Check sheet for the modelled part. Datum: model origin and axes. Units: mm. Face numbers are marked on the shaded views. A direction names the side the tool comes from. Give positions to 0.01 mm unless a question says otherwise; leave off trailing zeros. Loops run counter-clockwise (first coordinate to the right, second up) from the corner with the lowest first, then second, coordinate; pieces in that order, holes last. Notation, with made-up numbers: M 20,-1.5 L 54,-1.5 A17 ccw 54,8.5 Z; hole C -5,21.5 d10. An arc over 180 degrees is marked long. Use one line per item in the form item = value.
Autodesk Inventor part; units mm, degrees
ref_plane "Work Plane1" through (30.1625, 0, 0) normal (0, 0, -1) x (1, 0, 0)
ref_plane "YZ Plane" through (0, 0, 0) normal (1, 0, 0) x (0, 1, 0)
ref_plane "XZ Plane" through (0, 0, 0) normal (0, 1, 0) x (-1, 0, 0)
sketch "Sketch1" plane through (0, 0, 0) normal (0, 0, 1) x (1, 0, 0)
  line L0 (-3.3, 0) -> (50, 0)
  line L1 (50, 0) -> (50, 2.5)
  line L2 (50, 2.5) -> (12, 2.5)
  line L3 (12, 2.5) -> (11.5091, 2.2835)
  line L4 (11.5091, 2.2835) -> (0, 2.2835)
  line L5 (0, 2.2835) -> (0, 4.25)
  line L6 (-13.96, 0) -> (60.66, 0)
  line L7 (0, -0.85) -> (0, 5.1)
  line L8 (-3.3, 0) -> (-3.3, 3.9613)
  line L9 (0, 4.25) -> (-3.3, 3.9613)
  line L10 (12, 2.5) -> (0, 2.5) construction
  dimension "d0" = 50
  dimension "d1" = 38
  dimension "d2" = 0.4909
  dimension "d3" = 3.3
  dimension "d4" = 5
  dimension "d5" = 4.567
  dimension "d9" = 8.5
  dimension "d10" = 5
revolve "Body" add sketch "Sketch1" angle 360 about axis through (-3.3, 0, 0) along (1, 0, 0)
sketch "Sketch2" plane through (-3.3, 0, 0) normal (-1, 0, 0) x (0, 0, 1)
  circle A0 centre (0, 0) radius 4.25
  line L0 (0, 0) -> (0, 3.9613)
  line L1 (-4.25, 0.6) -> (4.25, 0.6)
  line L2 (4.25, 0.6) -> (4.25, -0.6)
  line L3 (4.25, -0.6) -> (-4.25, -0.6)
  line L4 (-4.25, -0.6) -> (-4.25, 0.6)
  line L5 (-4.25, 0) -> (4.25, 0) construction
  line L6 (0, 0.6) -> (0, -0.6) construction
  point P0 (0, 0)
  dimension "d11" = 1.2
  dimension "d12" = 8.5
fillet "Fillet1" radius 0.2 1 edges at (-3.3, -3.9613, 0)
extrude "Slot" cut sketch "Sketch2" against normal blind 1.3 contours A0 L3 L1 | L2 L3 A0 | A0 L1 L2 | A0 L4 L1 | L3 L4 A0
thread "Thread"
chamfer "Chamfer1" distance 0.433 distance2 0.4909 1 edges at (50, -2.5, 0) measured on face at (50, -0.4809, -0.0271)
ref_plane "Work Plane1" through (30.1625, 0, 0) normal (0, 0, -1) x (1, 0, 0)
equation "\"d11\" = SBR"
equation "\"d12\" = KOD"
equation "\"d14\" = RR"
equation "\"d19\" = STI"
equation "\"d15\" = GEL"
equation "\"d17\" = -0.5 * SPD + 0.5 * GD"
equation "\"d0\" = NLG"
equation "\"d1\" = GEL"
equation "\"d3\" = KOH"
equation "\"d4\" = GD"
equation "\"d5\" = BDM"
equation "\"d9\" = KOD"
equation "\"d10\" = KEWI"
equation "\"GD\" = 5"
equation "\"NLG\" = 50"
equation "\"GEL\" = 38"
equation "\"KOD\" = 8.5"
equation "\"KOH\" = 3.3"
equation "\"GAL\" = 0.61345 * PTC"
equation "\"SPD\" = 4.13397"
equation "\"BDM\" = 4.56699"
equation "\"GUL\" = 0.61345 * PTC"
equation "\"RR\" = 0.2"
equation "\"SBR\" = 1.2"
equation "\"STI\" = 1.3"
equation "\"KEWI\" = 5deg"
equation "\"PTC\" = 0.8"
equation "\"THREADDIA\" = 5"
equation "\"TOA\" = 30deg"
equation "\"NND\" = 5"
equation "\"GD1\" = THREADDIA - 1.2269 * PTC"
properties part number "DIN 84 - M5 x 50" material "Steel, Mild"
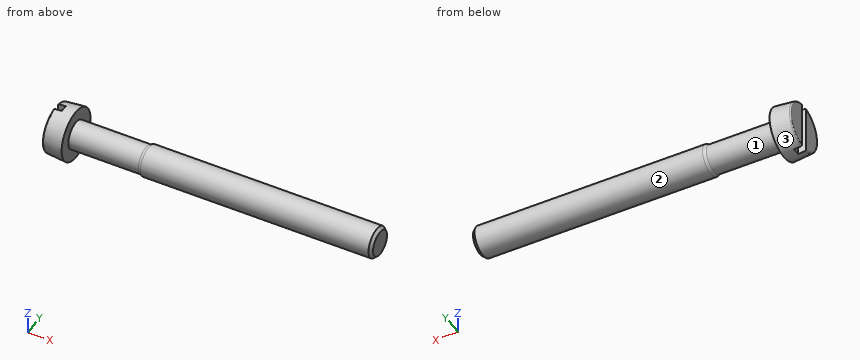
1) Section check C-C (x = 7). Record the cut outline in (y, z), then the cut area to 3 significant figures.
Evaluation:
outline = C 0,0 d4.57
area = 16.4 mm^2
2) Section check B-B (z = 0). Record the cut outline in (x, y).
Evaluation:
outline = M -3.3,-3.78 A0.2 ccw -3.12,-3.98 L 0,-4.25 L 0,-2.28 L 11.51,-2.28 L 12,-2.5 L 49.51,-2.5 L 50,-2.07 L 50,2.07 L 49.51,2.5 L 12,2.5 L 11.51,2.28 L 0,2.28 L 0,4.25 L -3.12,3.98 A0.2 ccw -3.3,3.78 L -3.3,0.6 L -2,0.6 L -2,-0.6 L -3.3,-0.6 Z
3) Set-up check for the marked faces 1, 2 and 3: record each of +Z, -Z, +X, -X, +Y, -Y from which the full face is reachable in a straight line by a thin tool's end or side.
Evaluation:
face_1 = none
face_2 = +X
face_3 = -X
4) Depth check by flat-ended pin: pin 1 Ø1.4 at (x, z) = (-3, 1) entering from -Y; pin 2 Ø5 at (x, z) = (44.5, 0) entering from +Y; pin 3 Ø3 at (x, y) = (17, 2) entering from -Z. Enter the tip coordinate at first touch or a pass-through.
Evaluation:
pin_1 = -4
pin_2 = 2.5
pin_3 = -2.45
5) Section check A-A (y = 0). Record the cut outline in (x, z), then the cut area to 3 significant figures.
Evaluation:
outline = M -2,-4.08 L 0,-4.25 L 0,-2.28 L 11.51,-2.28 L 12,-2.5 L 49.51,-2.5 L 50,-2.07 L 50,2.07 L 49.51,2.5 L 12,2.5 L 11.51,2.28 L 0,2.28 L 0,4.25 L -2,4.08 Z
area = 261 mm^2
6) Scan lines: line 1 (X direction, y = 1.5, z = -2.25); line 2 (X direction, y = 0.5, z = 3.25); line 3 (Z direction, x = 42, y = -1.75). Record each from-to range of solid material in increasing order.
Evaluation:
line_1 = -3.3 to 0
line_2 = -2 to 0
line_3 = -1.79 to 1.79
7) Section check D-D (x = 42.5). Record the cut outline in (y, z), then the cut area to 3 significant figures.
Evaluation:
outline = C 0,0 d5
area = 19.6 mm^2
